from build123d import *

# Parameters (mm, degrees)
SKETCH1_W           = 320.802
SKETCH1_H           = 438.15
BOSS_EXTRUDE1_DEPTH = 3.175
SKETCH2_R           = 13.97
SKETCH2_R_2         = 2.54
CUT_EXTRUDE1_DEPTH  = 3.175
SKETCH3_R           = 10.16
CUT_EXTRUDE3_DEPTH  = 3.175
SKETCH4_R           = 2.667
CUT_EXTRUDE4_DEPTH  = 3.175
SKETCH5_R           = 13.97
CUT_EXTRUDE5_DEPTH  = 3.175


with BuildPart() as part:
    # Sketch1 → Boss-Extrude1 (new body)
    with BuildSketch(Plane.XY):
        Rectangle(SKETCH1_W, SKETCH1_H)
    extrude(amount=BOSS_EXTRUDE1_DEPTH)

    # Sketch2 → Cut-Extrude1 (cut)
    with BuildSketch(Plane.XY.offset(3.175)):
        with Locations((106.445821197, -187.325)):
            Circle(SKETCH2_R)
        with Locations((55.626, -180.975)):
            Circle(SKETCH2_R)
        with Locations((4.826, -149.225)):
            Circle(SKETCH2_R)
        with Locations((-45.974, -142.875)):
            Circle(SKETCH2_R)
        with Locations((-96.774, -136.525)):
            Circle(SKETCH2_R)
        with Locations((106.445821197, 3.175)):
            Circle(SKETCH2_R)
        with Locations((106.445821197, 104.775)):
            Circle(SKETCH2_R)
        with Locations((93.745821197, 130.175)):
            Circle(SKETCH2_R_2)
        with Locations((106.445821197, 130.175)):
            Circle(SKETCH2_R_2)
        with Locations((119.145821197, 130.175)):
            Circle(SKETCH2_R_2)
        with Locations((93.745821197, 79.375)):
            Circle(SKETCH2_R_2)
        with Locations((106.445821197, 79.375)):
            Circle(SKETCH2_R_2)
        with Locations((119.145821197, 79.375)):
            Circle(SKETCH2_R_2)
    extrude(amount=-CUT_EXTRUDE1_DEPTH, mode=Mode.SUBTRACT)

    # Sketch3 → Cut-Extrude3 (cut)
    with BuildSketch(Plane.XY.offset(3.175)):
        with Locations((-99.314, 147.193)):
            Circle(SKETCH3_R)
        with Locations((-61.722, -87.757)):
            Circle(SKETCH3_R)
        with Locations((-99.314, -94.107)):
            Circle(SKETCH3_R)
    extrude(amount=-CUT_EXTRUDE3_DEPTH, mode=Mode.SUBTRACT)

    # Sketch4 → Cut-Extrude4 (cut)
    with BuildSketch(Plane.XY.offset(3.175)):
        with Locations((-147.701, -206.481352377)):
            Circle(SKETCH4_R)
        with Locations((-147.701, -193.781352377)):
            Circle(SKETCH4_R)
        with Locations((-147.701, -181.081352377)):
            Circle(SKETCH4_R)
        with Locations((-147.701, -168.381352377)):
            Circle(SKETCH4_R)
        with Locations((-147.701, -155.681352377)):
            Circle(SKETCH4_R)
        with Locations(Location((-147.701, 206.481352377, 0), (0, 0, 180))):
            Circle(SKETCH4_R)
        with Locations(Location((-147.701, 193.781352377, 0), (0, 0, 180))):
            Circle(SKETCH4_R)
        with Locations(Location((-147.701, 181.081352377, 0), (0, 0, 180))):
            Circle(SKETCH4_R)
        with Locations(Location((-147.701, 168.381352377, 0), (0, 0, 180))):
            Circle(SKETCH4_R)
        with Locations(Location((-147.701, 155.681352377, 0), (0, 0, 180))):
            Circle(SKETCH4_R)
        with Locations((147.701, 155.681352377)):
            Circle(SKETCH4_R)
        with Locations((147.701, 168.381352377)):
            Circle(SKETCH4_R)
        with Locations((147.701, 181.081352377)):
            Circle(SKETCH4_R)
        with Locations((147.701, 193.781352377)):
            Circle(SKETCH4_R)
        with Locations((147.701, 206.481352377)):
            Circle(SKETCH4_R)
        with Locations((147.701, 142.981352377)):
            Circle(SKETCH4_R)
        with Locations((147.701, 130.281352377)):
            Circle(SKETCH4_R)
        with Locations((147.701, 117.581352377)):
            Circle(SKETCH4_R)
        with Locations((147.701, 104.881352377)):
            Circle(SKETCH4_R)
        with Locations((147.701, 92.181352377)):
            Circle(SKETCH4_R)
        with Locations((147.701, 79.481352377)):
            Circle(SKETCH4_R)
        with Locations((147.701, 66.781352377)):
            Circle(SKETCH4_R)
        with Locations((147.701, 54.081352377)):
            Circle(SKETCH4_R)
        with Locations((147.701, 41.381352377)):
            Circle(SKETCH4_R)
        with Locations((147.701, 28.681352377)):
            Circle(SKETCH4_R)
        with Locations((147.701, 15.981352377)):
            Circle(SKETCH4_R)
        with Locations((147.701, 3.281352377)):
            Circle(SKETCH4_R)
        with Locations((147.701, -9.418647623)):
            Circle(SKETCH4_R)
        with Locations((147.701, -22.118647623)):
            Circle(SKETCH4_R)
        with Locations((147.701, -34.818647623)):
            Circle(SKETCH4_R)
        with Locations((147.701, -47.518647623)):
            Circle(SKETCH4_R)
        with Locations((147.701, -60.218647623)):
            Circle(SKETCH4_R)
        with Locations((147.701, -72.918647623)):
            Circle(SKETCH4_R)
        with Locations((147.701, -85.618647623)):
            Circle(SKETCH4_R)
        with Locations((147.701, -98.318647623)):
            Circle(SKETCH4_R)
        with Locations((147.701, -111.018647623)):
            Circle(SKETCH4_R)
        with Locations((147.701, -123.718647623)):
            Circle(SKETCH4_R)
        with Locations((147.701, -136.418647623)):
            Circle(SKETCH4_R)
        with Locations((147.701, -149.118647623)):
            Circle(SKETCH4_R)
        with Locations((147.701, -161.818647623)):
            Circle(SKETCH4_R)
        with Locations((147.701, -174.518647623)):
            Circle(SKETCH4_R)
        with Locations((147.701, -187.218647623)):
            Circle(SKETCH4_R)
        with Locations((147.701, -199.918647623)):
            Circle(SKETCH4_R)
        with Locations(Location((103.251, -206.481352377, 0), (0, 0, 180))):
            Circle(SKETCH4_R)
        with Locations(Location((115.951, -206.481352377, 0), (0, 0, 180))):
            Circle(SKETCH4_R)
        with Locations(Location((128.651, -206.481352377, 0), (0, 0, 180))):
            Circle(SKETCH4_R)
        with Locations(Location((90.551, -206.481352377, 0), (0, 0, 180))):
            Circle(SKETCH4_R)
        with Locations(Location((65.151, -206.481352377, 0), (0, 0, 180))):
            Circle(SKETCH4_R)
        with Locations(Location((77.851, -206.481352377, 0), (0, 0, 180))):
            Circle(SKETCH4_R)
        with Locations(Location((52.451, -206.481352377, 0), (0, 0, 180))):
            Circle(SKETCH4_R)
        with Locations(Location((39.751, -206.481352377, 0), (0, 0, 180))):
            Circle(SKETCH4_R)
        with Locations(Location((27.051, -206.481352377, 0), (0, 0, 180))):
            Circle(SKETCH4_R)
        with Locations(Location((14.351, -206.481352377, 0), (0, 0, 180))):
            Circle(SKETCH4_R)
        with Locations(Location((1.651, -206.481352377, 0), (0, 0, 180))):
            Circle(SKETCH4_R)
        with Locations(Location((-11.049, -206.481352377, 0), (0, 0, 180))):
            Circle(SKETCH4_R)
    extrude(amount=-CUT_EXTRUDE4_DEPTH, mode=Mode.SUBTRACT)

    # Sketch5 → Cut-Extrude5 (cut)
    with BuildSketch(Plane.XY.offset(3.175)):
        with Locations((-122.301, -48.514)):
            Circle(SKETCH5_R)
    extrude(amount=-CUT_EXTRUDE5_DEPTH, mode=Mode.SUBTRACT)


solid = part.part
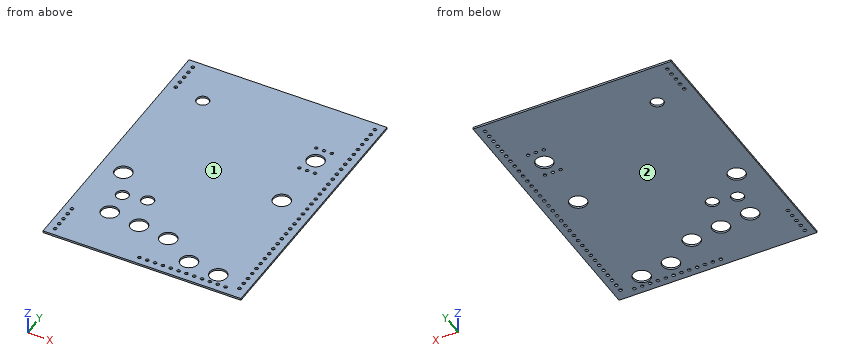
Geometry: final body of the model. Coordinates: model frame, mm. Face numbers are marked on the shaded views. Give positions to 0.01 mm unless a question says otherwise; leave off trailing zeros. Put each result on its own line as item: value.
Q1. Draft query along Z for the marked faces 1 and 2. Return one class per face: released by +Z, released by -Z, zero draft, split by the parting line, or undercut.
Here are the results:
face 1: released by +Z
face 2: released by -Z
Q2. Material intervals for L1, parallel to X at y = 130, z = 1.7; L2, parallel to X at y = 195, z = 2.45; L3, parallel to Y at x = -122, z = 2.9 (3 decimals), sorted ascending.
Here are the results:
L1: x = -160.4 to 91.21, 96.28 to 103.91, 108.98 to 116.61, 121.68 to 145.05, 150.35 to 160.4
L2: x = -160.4 to -150.07, -145.33 to 145.33, 150.07 to 160.4
L3: y = -219.075 to -62.481, -34.547 to 219.075
Q3. Section A-A, the plane z = 0.85. Count the separate pieces of the cut face and the enclosed holes in it, then the cut area to 3 significant figures.
Here are the results:
separate pieces: 1
enclosed holes: 72
area: 133,000 mm^2
Q4. Pin query (flat end, axial travel): pin 1 (7 mm diameter, centred on x = 90.55, y = -206.48, fed in from -Z). Return the tip coordinate at first contact, or that it passes through.
Here are the results:
pin 1: stops at z = 0
